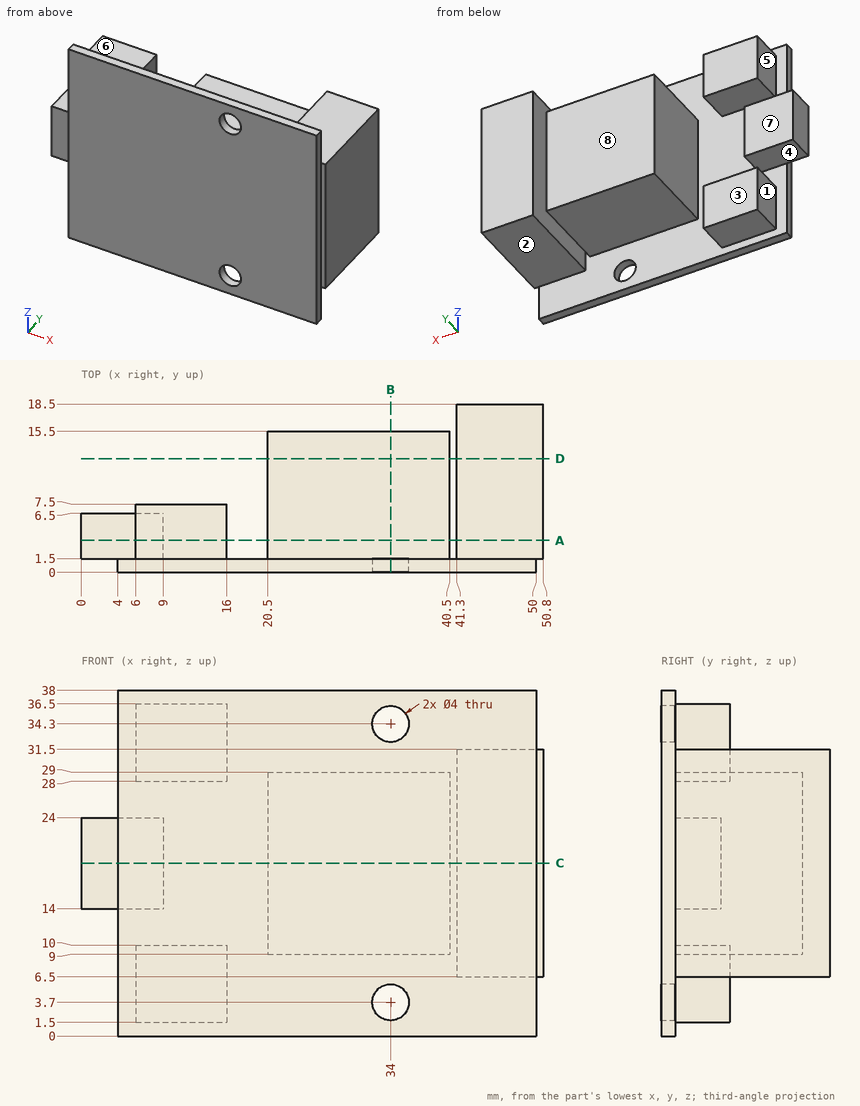
Answer from the drawing. Dimensions are ordinates in mm from the lowest x, y and z of the part. A direction names the side the tool comes from. Round coordinates to 2 decimals unless told otherwise and drop trailing zeros. Write each loop counter-clockwise with the first axis right and the second up, starting at its lowest first coordinate (ties: lowest second). Pieces come first, ordered by that corner, then holes. Notation, with made-up numbers: M -29.5,-30 L -0.5,-30 A23 ccw -0.5,-8 Z; hole C 68.5,48.5 d10. An arc over 180 degrees is marked long. Write each question's results on one line, items separated by ' | '. Start each with the question number.
Item 1: Find section C-C on z = 19. Write down the section's boundary in (x, y).
Item 2: Straight lines are drawn through the part: probe 1 along Z at (x, y) = (34, 0.85); probe 2 along X at (y, z) = (5.75, 19); probe 3 along X at (y, z) = (0.8, 34.3). For each, find the intervals that lie inside material, in ascending order.
Item 3: Find section B-B on x = 34. Write down the section's boundary in (y, z), and give its area (3 significant figures).
Item 4: Given pin 1 Ø2.5 at (x, z) = (9, 6.5) entering from +Y; pin 2 Ø6 at (x, z) = (38, 9) entering from +Y; pin 3 Ø3 at (x, y) = (11, 4) entering from -Z, each flat-ended and moving along its own axis, determine where each tip first touches the part or whether it passes through.
Item 5: The mould has two halves that part along Z. Classify the marked faces 6, 7 and 8: +Z half, -Z half, draft (parallel to the pull), parting line (faces both ways), or undercut.
Item 6: Find section D-D on y = 12.5. Write down the section's boundary in (x, z).
Item 7: Find section A-A on y = 3.5. Write down the section's boundary in (x, z).
Item 8: Which of the six approach directions +Z, -Z, +X, -X, +Y, -Y give full straight-line access (tool end or side, diameter ignored) to the marked faces 1, 2, 3, 4 and 5?
Answer block:
1) outline: M 0,1.5 L 4,1.5 L 4,0 L 50,0 L 50,1.5 L 50.8,1.5 L 50.8,18.5 L 41.3,18.5 L 41.3,1.5 L 40.5,1.5 L 40.5,15.5 L 20.5,15.5 L 20.5,1.5 L 9,1.5 L 9,6.5 L 0,6.5 Z
2) probe 1: z = 0 to 1.7, 5.7 to 32.3, 36.3 to 38 | probe 2: x = 0 to 9, 20.5 to 40.5, 41.3 to 50.8 | probe 3: x = 4 to 32, 36 to 50
3) outline: M 0,0 L 1.5,0 L 1.5,1.7 L 0,1.7 Z; M 0,5.7 L 1.5,5.7 L 1.5,9 L 15.5,9 L 15.5,29 L 1.5,29 L 1.5,32.3 L 0,32.3 Z; M 0,36.3 L 1.5,36.3 L 1.5,38 L 0,38 Z | area: 325 mm²
4) pin 1: stops at y = 7.5 | pin 2: stops at y = 15.5 | pin 3: stops at z = 1.5
5) face 6: +Z half | face 7: undercut | face 8: draft
6) outline: M 20.5,9 L 40.5,9 L 40.5,29 L 20.5,29 Z; M 41.3,6.5 L 50.8,6.5 L 50.8,31.5 L 41.3,31.5 Z
7) outline: M 0,14 L 9,14 L 9,24 L 0,24 Z; M 6,1.5 L 16,1.5 L 16,10 L 6,10 Z; M 6,28 L 16,28 L 16,36.5 L 6,36.5 Z; M 20.5,9 L 40.5,9 L 40.5,29 L 20.5,29 Z; M 41.3,6.5 L 50.8,6.5 L 50.8,31.5 L 41.3,31.5 Z
8) face 1: -Z, -X, +Y | face 2: -Z, +X, +Y | face 3: +Z, -Z, -X, +Y | face 4: -X, +Y | face 5: +Z, -X, +Y
